Geometry check sheet. Reference: the model listing, model coordinates, mm. A direction names the side the tool comes from. Round coordinates to 2 decimals unless told otherwise and drop trailing zeros. Order: outer loops, then holes, each group sorted by start corner. A loop starts at its lowest first (then second) coordinate and runs counter-clockwise, first axis right, second up. Notation, with made-up numbers: (56.25, 48.25) -> (77.25, 48.25) arc R21 ccw to (77.25, 87.25) -> close; hole circle Ø6 at (-10.75, 61). An arc over 180 degrees is marked (long way). Answer as a JSON object with one key per item and string values. Group by question number.
from build123d import *

# Parameters (mm, degrees)
BOSS_EXTRUDE1_DEPTH = 20
SKETCH2_R           = 43.5
CUT_EXTRUDE2_DEPTH  = 81.006249756
SKETCH3_R           = 47.5
CUT_EXTRUDE3_DEPTH  = 8
SKETCH4_R           = 6.5
CUT_EXTRUDE4_DEPTH  = 10
SKETCH4_3_R         = 5
CUT_EXTRUDE6_DEPTH  = 81.006249756


with BuildPart() as part:
    # Sketch1 → Boss-Extrude1 (new body)
    with BuildSketch(Plane(origin=(0, 0, 0), x_dir=(1, 0, 0), z_dir=(0, 1, 0))):
        with BuildLine():
            Line((-49, 34.626579386), (-49, 0))
            Line((-49, 0), (49, 0))
            Line((49, 0), (49, 34.626579386))
            ThreePointArc((49, 34.626579386), (0, 60), (-49, 34.626579386))
        make_face()
    extrude(amount=BOSS_EXTRUDE1_DEPTH)

    # Sketch2 → Cut-Extrude2 (cut, through all)
    with BuildSketch(Plane.XZ):
        Circle(SKETCH2_R)
    extrude(amount=-CUT_EXTRUDE2_DEPTH, mode=Mode.SUBTRACT)

    # Sketch3 → Cut-Extrude3 (cut)
    with BuildSketch(Plane(origin=(0, 20, 0), x_dir=(1, 0, 0), z_dir=(0, 1, 0))):
        Circle(SKETCH3_R)
    extrude(amount=-CUT_EXTRUDE3_DEPTH, mode=Mode.SUBTRACT)

    # Sketch4 → Cut-Extrude4 (cut)
    with BuildSketch(Plane.XZ):
        with Locations((38.183766184, -38.183766184)):
            Circle(SKETCH4_R)
        with Locations((-38.183766184, -38.183766184)):
            Circle(SKETCH4_R)
    extrude(amount=-CUT_EXTRUDE4_DEPTH, mode=Mode.SUBTRACT)

    # Sketch4_3 → Cut-Extrude6 (cut, through all)
    with BuildSketch(Plane.XZ):
        with Locations((-38.183766184, 38.183766184)):
            Circle(SKETCH4_3_R)
        with Locations((38.183766184, 38.183766184)):
            Circle(SKETCH4_3_R)
        with Locations(Location((38.183766184, -38.183766184, 0), (0, 0, 270))):
            Circle(SKETCH4_3_R)
        with Locations(Location((-38.183766184, -38.183766184, 0), (0, 0, 270))):
            Circle(SKETCH4_3_R)
    extrude(amount=-CUT_EXTRUDE6_DEPTH, mode=Mode.SUBTRACT)


solid = part.part
Item 1: Set-up check for faces 1 (the flat face through (49, 10, -17)), 2 (the cylindrical face through (1.04, 16.06, -47.49)), 3 (the flat face through (-37, 10, -33)): record each of +Z, -Z, +X, -X, +Y, -Y from which the full face is reachable in a straight line by a thin tool's end or side.
Item 2: Depth check by flat-ended pin: pin 1 Ø8 at (x, y) = (-3, 3.5) entering from +Z; pin 2 Ø4 at (y, z) = (10, -45) entering from +X; pin 3 Ø11.5 at (x, z) = (38.18, -38.18) entering from -Y. Enter the tip coordinate at first touch or a pass-through.
Item 3: Sectioned sample at C-C, the plane z = -10.5. Enter the section's corners in (x, y).
Item 4: Sectioned sample at B-B, the plane x = 0. Enter the section's corners in (y, z).
Item 5: Sectioned sample at A-A, the plane z = -39.5. Enter the section's corners in (x, y).
Item 6: Mould release check, pull along X, two halves, no side actions. Record for faces 4 (the cylindrical face through (0.803, 9.86, -59.995)), 5 (the cylindrical face through (33.766, 4.93, -33.416)), 6 (the flat face through (-4, 0, -46)): pulls with the +X half, pulls with the -X half, needs draft (parallel to the pull), parting line crosses it, or undercut.
Item 7: Sectioned sample at D-D, the plane y = 14.25. Enter the section's corners in (x, z).
Item 8: Thickness scan on L1, parallel to X at y = 11, z = -35; L2, parallel to X at y = 16.5, z = -40.5; L3, parallel to X at y = 7, z = -9.5. Record the ranges inside material, lowest first.
Result:
{
 "1": {"face 1": "+Z, -Z, +X, +Y, -Y", "face 2": "+Z, +Y", "face 3": "-Y"},
 "2": {"pin 1": "stops at z = -42.93", "pin 2": "stops at x = 41.84", "pin 3": "stops at y = 10"},
 "3": {"outline": "(-49, 0) -> (-42.21, 0) -> (-42.21, 12) -> (-46.32, 12) -> (-46.32, 20) -> (-49, 20) -> close; (42.21, 0) -> (49, 0) -> (49, 20) -> (46.32, 20) -> (46.32, 12) -> (42.21, 12) -> close"},
 "4": {"outline": "(0, -60) -> (20, -60) -> (20, -47.5) -> (12, -47.5) -> (12, -43.5) -> (0, -43.5) -> close"},
 "5": {"outline": "(-45.16, 0) -> (-44.55, 0) -> (-44.55, 10) -> (-43.01, 10) -> (-43.01, 20) -> (-45.16, 20) -> close; (-33.36, 10) -> (-31.82, 10) -> (-31.82, 0) -> (-18.22, 0) -> (-18.22, 12) -> (-26.38, 12) -> (-26.38, 20) -> (-33.36, 20) -> close; (18.22, 0) -> (31.82, 0) -> (31.82, 10) -> (33.36, 10) -> (33.36, 20) -> (26.38, 20) -> (26.38, 12) -> (18.22, 12) -> close; (43.01, 10) -> (44.55, 10) -> (44.55, 0) -> (45.16, 0) -> (45.16, 20) -> (43.01, 20) -> close"},
 "6": {"face 4": "parting line crosses it", "face 5": "undercut", "face 6": "needs draft"},
 "7": {"outline": "(-49, -34.63) arc R60 ccw to (49, -34.63) -> (49, 0) -> (47.5, 0) arc R47.5 cw to (-47.5, 0) -> (-49, 0) -> close; hole circle Ø10 at (-38.18, -38.18); hole circle Ø10 at (38.18, -38.18)"},
 "8": {"L1": "x = -48.73 to -42.04, -34.33 to -25.83, 25.83 to 34.33, 42.04 to 48.73", "L2": "x = -44.27 to -42.61, -33.75 to -24.82, 24.82 to 33.75, 42.61 to 44.27", "L3": "x = -49 to -42.45, 42.45 to 49"}
}
